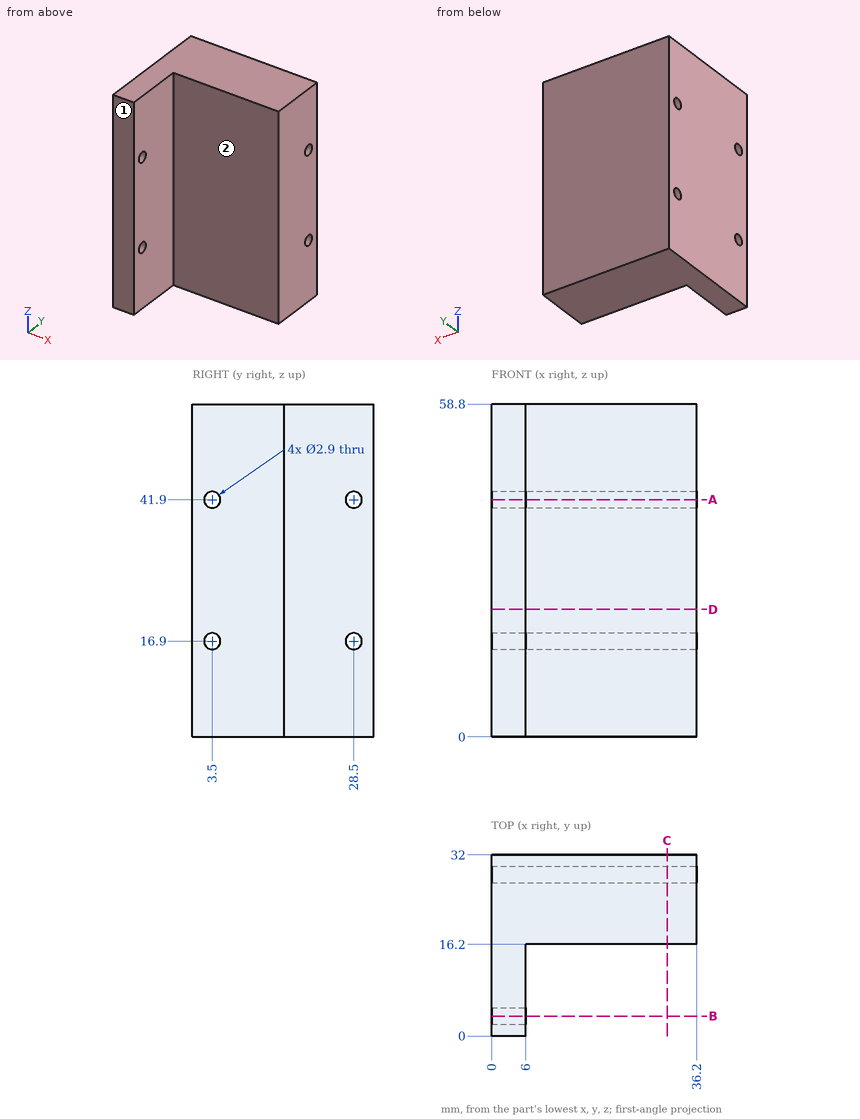
Here's the drawing with two shaded views (mm, measured from the low corner). I have some questions. A direction names the side the tool comes from. Round coordinates to 2 decimals unless told otherwise and drop trailing zeros. Write each loop counter-clockwise with the first axis right and the second up, starting at its lowest first coordinate (ties: lowest second). Pieces come first, ordered by that corner, then holes. Notation, with made-up numbers: M 73,25 L 120,25 A14 cw 120,52 Z; hole C 11,21 d7. An arc over 180 degrees is marked long. Answer in a Markdown table with one row per item. Add a question column.
Q1. Imagine slicing it at D-D (z = 22.5). Please give me the cut outline in (x, y), then the cut area to 3 significant figures.
Q2. Imagine slicing it at C-C (x = 31). Please give me the cut outline in (y, z).
Q3. On a 3-axis mill with a long thin cutter (end or side, diameter ignored), from which of +Z, -Z, +X, -X, +Y, -Y can I reach the whole of each face in a straight line? I mean the marked faces 1 and 2. Say none if no direction works.
Q4. Imagine slicing it at B-B (y = 3.5). Please give me the cut outline in (x, z).
Q5. If I drill on line 1 (Y direction, x = 2.2, z = 16.9); line 2 (Z direction, x = 26, y = 28); line 3 (X direction, y = 3, z = 39.5), over which ranges is the centre line in solid material (lowest first)? Write a range as from..to.
Q6. Will these pins go through, and if not, where does the flat tip stop? pin 1 Ø3.5 at (y, z) = (28.5, 16.9) entering from +X; pin 2 Ø2 at (y, z) = (5, 24) entering from +X; pin 3 Ø6 at (x, y) = (28, 12.5) entering from +Z; pin 4 Ø2 at (x, z) = (31.5, 44) entering from -Y.
Q7. Imagine slicing it at A-A (z = 41.9). Please give me the cut outline in (x, y), then the cut area to 3 significant figures.
Values:
| question | item | result |
|---|---|---|
| 1 | outline | M 0,0 L 6,0 L 6,16.2 L 36.2,16.2 L 36.2,32 L 0,32 Z |
| 1 | area | 669 mm^2 |
| 2 | outline | M 16.2,0 L 32,0 L 32,58.8 L 16.2,58.8 Z; hole C 28.5,16.9 d2.9; hole C 28.5,41.9 d2.9 |
| 3 | face 1 | +Z, -Z, +X, -X, -Y |
| 3 | face 2 | +Z, -Z, +X, -Y |
| 4 | outline | M 0,0 L 6,0 L 6,15.45 L 0,15.45 Z; M 0,18.35 L 6,18.35 L 6,40.45 L 0,40.45 Z; M 0,43.35 L 6,43.35 L 6,58.8 L 0,58.8 Z |
| 5 | line 1 | 0..2.05, 4.95..27.05, 29.95..32 |
| 5 | line 2 | 0..15.54, 18.26..40.54, 43.26..58.8 |
| 5 | line 3 | 0..6 |
| 6 | pin 1 | x = 36.2 |
| 6 | pin 2 | x = 6 |
| 6 | pin 3 | through |
| 6 | pin 4 | y = 16.2 |
| 7 | outline | M 0,0 L 6,0 L 6,2.05 L 0,2.05 Z; M 0,4.95 L 6,4.95 L 6,16.2 L 36.2,16.2 L 36.2,27.05 L 0,27.05 Z; M 0,29.95 L 36.2,29.95 L 36.2,32 L 0,32 Z |
| 7 | area | 547 mm^2 |
